Check sheet for the modelled part. Datum: model origin and axes. Units: mm. Face numbers are marked on the shaded views. A direction names the side the tool comes from. Give positions to 0.01 mm unless a question says otherwise; leave off trailing zeros. Loops run counter-clockwise (first coordinate to the right, second up) from the corner with the lowest first, then second, coordinate; pieces in that order, holes last. Notation, with made-up numbers: (21, 47.25) - (73, 47.25) arc R25 cw to (73, 83.25) - close; hole circle Ø2 at (33, -33). An arc over 180 degrees is marked (long way). Use CSV: the item, a comma, the result in double quotes.
from build123d import *

# Parameters (mm, degrees)
F0_W     = 20
F0_H     = 50
F0_R     = 25
F0_H_2   = 30
F1_DEPTH = 100
F2_W     = 30
F2_H     = 60
F2_W_2   = 55.66628
F3_DEPTH = 100.001
F5_DEPTH = 60.001
F4_R     = 15
F6_DEPTH = 60.001


with BuildPart() as f1:
    # F0 (on Top) → F1 (new body)
    with BuildSketch(Plane.XY):
        with Locations((50, -55)):
            Rectangle(F0_W, F0_H)
        with BuildLine():
            Line((0, 50), (0, 0))
            Line((0, 0), (40, 0))
            Line((40, 0), (60, 0))
            Line((60, 0), (100, 0))
            Line((100, 0), (100, 50))
            ThreePointArc((100, 50), (50, 100), (0, 50))
        make_face()
        with Locations((50, 50)):
            Circle(F0_R, mode=Mode.SUBTRACT)
        with Locations((50, -15)):
            Rectangle(F0_W, F0_H_2)
    extrude(amount=-F1_DEPTH)

    # F2 (on face) → F3 (cut, through all)
    with BuildSketch(Plane(origin=(0, 0, 0), x_dir=(0, -1, 0), z_dir=(-1, 0, 0))):
        with Locations((-35, -49.526112)):
            Rectangle(F2_W, F2_H)
        with Locations((-77.83314, -49.526112)):
            Rectangle(F2_W_2, F2_H)
    extrude(amount=-F3_DEPTH, mode=Mode.SUBTRACT)

    # F4 (on face) → F5 (cut, through all)
    with BuildSketch(Plane(origin=(40, 0, 0), x_dir=(0, -1, 0), z_dir=(-1, 0, 0))):
        with BuildLine():
            Line((80, -100), (80, -50))
            ThreePointArc((80, -50), (65.355339, -85.355339), (30, -100))
            Line((30, -100), (80, -100))
        make_face()
        with BuildLine():
            Line((80, 0), (30, 0))
            ThreePointArc((30, 0), (65.355339, -14.644661), (80, -50))
            Line((80, -50), (80, 0))
        make_face()
    extrude(amount=-F5_DEPTH, mode=Mode.SUBTRACT)

    # F4 (on face) → F6 (cut, through all)
    with BuildSketch(Plane(origin=(40, 0, 0), x_dir=(0, -1, 0), z_dir=(-1, 0, 0))):
        with Locations((30, -50)):
            Circle(F4_R)
    extrude(amount=-F6_DEPTH, mode=Mode.SUBTRACT)


solid = f1.part
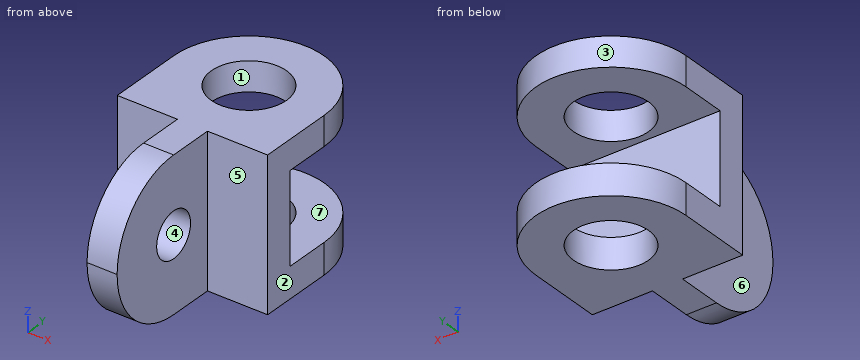
1. Set-up check for the marked faces 5, 6 and 7: record each of +Z, -Z, +X, -X, +Y, -Y from which the full face is reachable in a straight line by a thin tool's end or side.
Completed:
face 5,"+Z, -Z, +X, -Y"
face 6,"+Z, -Z, -X, -Y"
face 7,"+X, -X, +Y"
2. Sectioned sample at D-D, the plane z = -83.5. Record the boundary of the cut face in (x, y), and give its area (3 significant figures).
Completed:
outline,"(0, 0) - (40, 0) - (40, -67.12) - (60, -67.12) - (60, 0) - (100, 0) - (100, 50) arc R50 ccw to (0, 50) - close; hole circle Ø50 at (50, 50)"
area,"8,310 mm²"
3. Sectioned sample at A-A, the plane x = 50. Record the boundary of the cut face in (y, z).
Completed:
outline,"(-30, -100) - (25, -100) - (25, -79.53) - (20, -79.53) - (20, -19.53) - (25, -19.53) - (25, 0) - (-30, 0) arc R50 ccw to start; (75, -100) - (100, -100) - (100, -79.53) - (75, -79.53) - close; (75, -19.53) - (100, -19.53) - (100, 0) - (75, 0) - close; hole circle Ø30 at (-30, -50)"
4. Scan lines: line 1 along Z through (x, y) = (85.5, 50); line 2 along Z through (x, y) = (48, -30); line 3 along X through (y, z) = (-29, -92). Record each from-to range of solid material in increasing order.
Completed:
line 1,"z = -100 to -79.53, -19.53 to 0"
line 2,"z = -100 to -65, -35 to 0"
line 3,"x = 40 to 60"
5. Sectioned sample at B-B, the plane y = 63. Record the boundary of the cut face in (x, z).
Completed:
outline,"(1.72, -100) - (28.65, -100) - (28.65, -79.53) - (1.72, -79.53) - close; (1.72, -19.53) - (28.65, -19.53) - (28.65, 0) - (1.72, 0) - close; (71.35, -100) - (98.28, -100) - (98.28, -79.53) - (71.35, -79.53) - close; (71.35, -19.53) - (98.28, -19.53) - (98.28, 0) - (71.35, 0) - close"
6. Sectioned sample at C-C, the plane z = -58. Record the boundary of the cut face in (x, y).
Completed:
outline,"(0, 0) - (40, 0) - (40, -17.31) - (60, -17.31) - (60, 0) - (100, 0) - (100, 20) - (0, 20) - close; (40, -79.36) - (60, -79.36) - (60, -42.69) - (40, -42.69) - close"
7. Release check for a two-part mould opening along Y. For the marked faces 1, 2, 3 and 4 record: released by +Y, released by -Y, zero draft, split by the parting line, or undercut.
Completed:
face 1,"undercut"
face 2,"zero draft"
face 3,"released by +Y"
face 4,"undercut"
8. Go/stop test with flat-tipped pins: pin 1 Ø8 at (x, z) = (26, -81) entering from +Y; pin 2 Ø24 at (y, z) = (-40, -63.5) entering from +X; pin 3 Ø5 at (x, y) = (71, 38.5) entering from -Z; pin 4 Ø12 at (x, z) = (16.5, -61.5) entering from +Y. Record where each tip stops, or that it passes through.
Completed:
pin 1,"stops at y = 95.83"
pin 2,"stops at x = 60"
pin 3,"stops at z = -100"
pin 4,"stops at y = 20"
